from build123d import *

# Parameters (mm, degrees)
PAD002_DEPTH    = 4
SKETCH_W        = 100
SKETCH_H        = 150
PAD_DEPTH       = 4
POCKET_DEPTH    = 5
SKETCH002_R     = 6
POCKET001_DEPTH = 5
PAD001_DEPTH    = 4
PAD003_DEPTH    = 4


with BuildPart() as pad002:
    # Sketch004 → Pad002 (new body)
    with BuildSketch(Plane.XY):
        Polygon((-28.9324500821, 15), (-27.2459600657, 27), (-23.2459600657, 27), (-24.9324500821, 15), align=None)
        Polygon((13.7540399343, 27), (12.0675499179, 15), (8.0675499179, 15), (9.7540399343, 27), align=None)
        Polygon((-13.7540399343, 123), (-12.0675499179, 135), (-8.0675499179, 135), (-9.7540399343, 123), align=None)
        Polygon((28.9324500821, 135), (27.2459600657, 123), (23.2459600657, 123), (24.9324500821, 135), align=None)
    extrude(amount=PAD002_DEPTH)


with BuildPart() as pocket001:
    # Sketch → Pad (new body)
    with BuildSketch(Plane.XY):
        with Locations((0, 75)):
            Rectangle(SKETCH_W, SKETCH_H)
    extrude(amount=PAD_DEPTH)

    # Sketch001 → Pocket (cut)
    with BuildSketch(Plane.XY.offset(4)):
        with BuildLine():
            Line((-39.2459600657, 27), (-25.7540399343, 123))
            ThreePointArc((-11.9496190476, 135), (-21.0951375679, 131.5806307393), (-25.7540399343, 123))
            Line((-11.9496190476, 135), (28.8145192119, 135))
            ThreePointArc((39.2459600657, 123), (36.764597172, 131.3769407401), (28.8145192119, 135))
            Line((39.2459600657, 123), (25.7540399343, 27))
            ThreePointArc((11.9496190476, 15), (21.0951375679, 18.4193692607), (25.7540399343, 27))
            Line((-28.8145192119, 15), (11.9496190476, 15))
            ThreePointArc((-39.2459600657, 27), (-36.764597172, 18.6230592599), (-28.8145192119, 15))
        make_face()
    extrude(amount=-POCKET_DEPTH, mode=Mode.SUBTRACT)

    # Sketch002 → Pocket001 (cut)
    with BuildSketch(Plane.XY.offset(4)):
        with Locations((36, 21)):
            Circle(SKETCH002_R)
    extrude(amount=-POCKET001_DEPTH, mode=Mode.SUBTRACT)


with BuildPart() as pad001:
    # Sketch003 → Pad001 (new body)
    with BuildSketch(Plane.XY):
        Polygon((-27.2459600657, 27), (13.7540399343, 27), (19.6567549918, 69), (-21.3432450082, 69), align=None)
        Polygon((-13.7540399343, 123), (27.2459600657, 123), (21.3432450082, 81), (-19.6567549918, 81), align=None)
    extrude(amount=PAD001_DEPTH)


with BuildPart() as fusion:
    # Sketch005 → Pad003 (new body)
    with BuildSketch(Plane.XY):
        Polygon((-21.3432450082, 69), (-26.5589654351, 75), (-19.6567549918, 81), (-18.8082148769, 87.0376766418), (-30.3552409675, 77), (-32.3368492008, 77), (-32.8990125396, 73), (-30.1204439329, 73), (-22.0808696766, 63.7515277681), align=None)
        Polygon((21.3432450082, 81), (26.5589654351, 75), (19.6567549918, 69), (18.8082148769, 62.9623233582), (30.3552409675, 73), (32.3368492008, 73), (32.8990125396, 77), (30.1204439329, 77), (22.0808696766, 86.2484722319), align=None)
    extrude(amount=PAD003_DEPTH)

    # Fusion: union Pad002, Pocket001, Pad001
    add(pad002.part)
    add(pocket001.part)
    add(pad001.part)


solid = fusion.part
The model under review builds one solid part; all positions refer to its coordinate system, in mm. A direction names the side the tool comes from. Round coordinates to 2 decimals unless told otherwise and drop trailing zeros. Loops run counter-clockwise (first coordinate to the right, second up) from the corner with the lowest first, then second, coordinate; pieces in that order, holes last. Notation, with made-up numbers: (60, -16) -> (102, -16) arc R23 ccw to (102, -3) -> close; hole circle Ø11 at (-25, 16). An arc over 180 degrees is marked (long way). Write item = value, one per line. Start each with the question number.
Item 1: Insertion check: pin 1 (2 mm diameter, centred on x = 31.5, z = 1, fed in from -Y). The pin has a flat end and moves straight along its axis. Give the tip position at first contact, or say it passes through.
Item 2: For faces 1 (the flat face through (7, 123, 2)), 2 (the flat face through (50, 74, 2)), list the 3-axis set-ups (+Z, -Z, +X, -X, +Y, -Y) from which the entire face can be reached by the end or side of a thin tool; tool diameter is ignored.
Item 3: Take a section at D-D on z = 1.9. Count the separate pieces of the cut face and the enclosed holes in it, plus the area to 3 significant figures.
Item 4: Take a section at C-C on x = 16.5. Give the boundary of the cut face in (y, z), plus the area to 3 significant figures.
Item 5: Take a section at B-B on y = 132. Give the boundary of the cut face in (x, z).
Item 6: To check wall thickness, follow L1, parallel to X at y = 124, z = 0.55; L2, parallel to X at y = 44.5, z = 2.4; L3, parallel to X at y = 19.5, z = 0.6. State the ranges of each line that lie inside material, in increasing order.
Item 7: Take a section at A-A on y = 116. Give the boundary of the cut face in (x, z).
Item 8: Mouldability with a two-part tool opening along Y and no side actions: class faces 3 (the flat face through (1, 93, 4)), 4 (the flat face through (-7, 27, 2)) as released by +Y, released by -Y, zero draft, split by the parting line, or undercut.
Result:
q1.pin_1 = 0
q2.face_1 = +Z, -Z
q2.face_2 = +Z, -Z, +X, +Y, -Y
q3.separate_pieces = 1
q3.enclosed_holes = 8
q3.area = 11,100 mm²
q4.outline = (0, 0) -> (15.76, 0) -> (15.76, 4) -> (0, 4) -> close; (46.54, 0) -> (69, 0) -> (69, 4) -> (46.54, 4) -> close; (81, 0) -> (123, 0) -> (123, 4) -> (81, 4) -> close; (135, 0) -> (150, 0) -> (150, 4) -> (135, 4) -> close
q4.area = 381 mm²
q5.outline = (-50, 0) -> (-20.59, 0) -> (-20.59, 4) -> (-50, 4) -> close; (-12.49, 0) -> (-8.49, 0) -> (-8.49, 4) -> (-12.49, 4) -> close; (24.51, 0) -> (28.51, 0) -> (28.51, 4) -> (24.51, 4) -> close; (36.18, 0) -> (50, 0) -> (50, 4) -> (36.18, 4) -> close
q6.L1 = -50 to -25.58, -13.61 to -9.61, 23.39 to 27.39, 39.34 to 50
q6.L2 = -50 to -36.79, -24.79 to 16.21, 28.21 to 50
q6.L3 = -50 to -37.45, -28.3 to -24.3, 8.7 to 12.7, 22.21 to 30.19, 41.81 to 50
q7.outline = (-50, 0) -> (-26.74, 0) -> (-26.74, 4) -> (-50, 4) -> close; (-14.74, 0) -> (26.26, 0) -> (26.26, 4) -> (-14.74, 4) -> close; (38.26, 0) -> (50, 0) -> (50, 4) -> (38.26, 4) -> close
q8.face_3 = zero draft
q8.face_4 = undercut
